```python
from build123d import *

# Parameters (mm, degrees)
SKETCH_1_W          = 30
SKETCH_1_H          = 10
SKETCH_1_W_2        = 26
SKETCH_1_H_2        = 6
EXTRUDE_1_DEPTH     = 50
SKETCH_2_R          = 2
SKETCH_2_R_2        = 1.5
CUT_EXTRUDE_1_DEPTH = 54.150729064
SKETCH_3_R          = 1.5
CUT_EXTRUDE_2_DEPTH = 54.150729064
SKETCH_4_R          = 1.5
CUT_EXTRUDE_3_DEPTH = 59.523499554


with BuildPart() as part:
    # 草图1 → 凸台-拉伸1 (new, symmetric)
    with BuildSketch(Plane(origin=(0, 0, 0), x_dir=(1, 0, 0), z_dir=(0, 1, 0))):
        Rectangle(SKETCH_1_W, SKETCH_1_H)
        Rectangle(SKETCH_1_W_2, SKETCH_1_H_2, mode=Mode.SUBTRACT)
    extrude(amount=EXTRUDE_1_DEPTH, both=True)

    # 草图2 → 切除-拉伸1 (cut, through all)
    with BuildSketch(Plane(origin=(0, 0, -5), x_dir=(-1, 0, 0), z_dir=(0, 0, -1))):
        with Locations((2, 45)):
            Circle(SKETCH_2_R)
        with Locations((10, 45)):
            Circle(SKETCH_2_R_2)
        with Locations((-10, 45)):
            Circle(SKETCH_2_R_2)
        with Locations((-10, -45)):
            Circle(SKETCH_2_R_2)
        with Locations((2, -45)):
            Circle(SKETCH_2_R)
        with Locations((10, -45)):
            Circle(SKETCH_2_R_2)
    extrude(amount=-CUT_EXTRUDE_1_DEPTH, mode=Mode.SUBTRACT)

    # 草图3 → 切除-拉伸2 (cut, through all)
    with BuildSketch(Plane.XY.offset(5)):
        with Locations((0, -35)):
            Circle(SKETCH_3_R)
        with Locations((10, -35)):
            Circle(SKETCH_3_R)
        with Locations((-10, -35)):
            Circle(SKETCH_3_R)
    extrude(amount=-CUT_EXTRUDE_2_DEPTH, mode=Mode.SUBTRACT)

    # 草图4 → 切除-拉伸3 (cut, through all)
    with BuildSketch(Plane(origin=(15, 0, 0), x_dir=(0, 0, -1), z_dir=(1, 0, 0))):
        with Locations((0, 30)):
            Circle(SKETCH_4_R)
        Circle(SKETCH_4_R)
        with Locations((0, -30)):
            Circle(SKETCH_4_R)
    extrude(amount=-CUT_EXTRUDE_3_DEPTH, mode=Mode.SUBTRACT)


solid = part.part
```
Design review of the part built by this model. Coordinates are the model's own, in mm. A direction names the side the tool comes from. Coordinates: 2 decimals unless noted, no trailing zeros. Order: outer loops, then holes, each group sorted by start corner. A loop starts at its lowest first (then second) coordinate and runs counter-clockwise, first axis right, second up. Notation, with made-up numbers: (-2, 28.5) - (15, 28.5) arc R27 cw to (15, 63.5) - close; hole circle Ø4 at (77, 13.5). An arc over 180 degrees is marked (long way). Answer in a Markdown table with one row per item.
(1) The part is to be moulded in two halves that separate along X. For faces 3 (the cylindrical face through (14.014, -28.513, 0.195)), 4 (the flat face through (-15, 1, -2)), 5 (the cylindrical face through (-2, -47, 4)), say which applies: released by +X, released by -X, zero draft, split by the parting line, or undercut.
Checked values:
| item | result |
|---|---|
| face 3 | zero draft |
| face 4 | released by -X |
| face 5 | undercut |
(2) Wall thickness on line 1 along Z through (x, y) = (4, 34); line 2 along X through (y, z) = (-28.5, -2); line 3 along Y through (x, z) = (-13.35, 0): over which ranges is each line inside the solid? List them lowest first. Write a range as from..to.
Checked values:
| item | result |
|---|---|
| line 1 | -5..-3, 3..5 |
| line 2 | -15..-13, 13..15 |
| line 3 | -50..-31.5, -28.5..-1.5, 1.5..28.5, 31.5..50 |
(3) Consider section A-A on x = 3.5. State the section outline as (y, z) points.
Checked values:
| item | result |
|---|---|
| outline | (-50, -5) - (50, -5) - (50, -3) - (-50, -3) - close; (-50, 3) - (50, 3) - (50, 5) - (-50, 5) - close |
(4) Consider section B-B on y = -35. Give the number of separate pieces and of enclosed holes in the cut face, plus the area to 3 significant figures.
Checked values:
| item | result |
|---|---|
| separate pieces | 6 |
| enclosed holes | 0 |
| area | 108 mm^2 |
(5) For faces 1 (the flat face through (-13, 1, 2)), 2 (the flat face through (-0.2, 50, -3.4)), list the 3-axis set-ups (+Z, -Z, +X, -X, +Y, -Y) from which the entire face can be reached by the end or side of a thin tool; tool diameter is ignored.
Checked values:
| item | result |
|---|---|
| face 1 | +Y, -Y |
| face 2 | +Z, -Z, +X, -X, +Y |
